```python
from build123d import *

# Parameters (mm, degrees)
SKETCH_W        = 57
SKETCH_H        = 34
PAD_DEPTH       = 15
SKETCH001_W     = 53.5
SKETCH001_H     = 30.5
POCKET_DEPTH    = 2
SKETCH002_W     = 10
SKETCH002_H     = 15.25
POCKET001_DEPTH = 10.7
SKETCH003_W     = 10
SKETCH003_H     = 4.2
POCKET002_DEPTH = 0.45
SKETCH004_W     = 13
SKETCH004_H     = 11.05
POCKET003_DEPTH = 4.9
SKETCH005_W     = 8.9
SKETCH005_H     = 4
POCKET004_DEPTH = 3.6
SKETCH006_W     = 4.5
SKETCH006_H     = 2.4
POCKET005_DEPTH = 2.1
SKETCH007_W     = 51
SKETCH007_H     = 30.5
POCKET006_DEPTH = 2.5


with BuildPart() as part:
    # Sketch → Pad (new body)
    with BuildSketch(Plane.XY):
        Rectangle(SKETCH_W, SKETCH_H)
    extrude(amount=PAD_DEPTH)

    # Sketch001 (on Face6 of Pad) → Pocket (cut)
    with BuildSketch(Plane.XY.offset(15)):
        Rectangle(SKETCH001_W, SKETCH001_H)
    extrude(amount=-POCKET_DEPTH, mode=Mode.SUBTRACT)

    # Sketch002 (on Face11 of Pocket) → Pocket001 (cut)
    with BuildSketch(Plane.XY.offset(13)):
        with Locations((-19.75, 7.625)):
            Rectangle(SKETCH002_W, SKETCH002_H)
        with Locations((20.2, 7.625)):
            Rectangle(SKETCH002_W, SKETCH002_H)
    extrude(amount=-POCKET001_DEPTH, mode=Mode.SUBTRACT)

    # Sketch003 (on Face18 of Pocket001) → Pocket002 (cut)
    with BuildSketch(Plane.XY.offset(2.3)):
        with Locations((-19.75, 13.15)):
            Rectangle(SKETCH003_W, SKETCH003_H)
        with Locations((20.2, 13.15)):
            Rectangle(SKETCH003_W, SKETCH003_H)
    extrude(amount=-POCKET002_DEPTH, mode=Mode.SUBTRACT)

    # Sketch004 (on Face10 of Pocket002) → Pocket003 (cut)
    with BuildSketch(Plane.XY.offset(13)):
        with Locations((-7.8, 9.725)):
            Rectangle(SKETCH004_W, SKETCH004_H)
        with Locations((7.8, 9.725)):
            Rectangle(SKETCH004_W, SKETCH004_H)
    extrude(amount=-POCKET003_DEPTH, mode=Mode.SUBTRACT)

    # Sketch005 (on Face10 of Pocket003) → Pocket004 (cut)
    with BuildSketch(Plane.XY.offset(13)):
        with Locations((10.55, -0.3)):
            Rectangle(SKETCH005_W, SKETCH005_H)
    extrude(amount=-POCKET004_DEPTH, mode=Mode.SUBTRACT)

    # Sketch006 (on Face36 of Pocket004) → Pocket005 (cut)
    with BuildSketch(Plane.XY.offset(9.4)):
        with Locations((10.5, -0.3)):
            Rectangle(SKETCH006_W, SKETCH006_H)
    extrude(amount=-POCKET005_DEPTH, mode=Mode.SUBTRACT)

    # Sketch007 (on Face11 of Pocket005) → Pocket006 (cut)
    with BuildSketch(Plane.XY.offset(13)):
        Rectangle(SKETCH007_W, SKETCH007_H)
    extrude(amount=-POCKET006_DEPTH, mode=Mode.SUBTRACT)


solid = part.part
```
Geometry check sheet. Reference: the model listing, model coordinates, mm. A direction names the side the tool comes from. Round coordinates to 2 decimals unless told otherwise and drop trailing zeros. Order: outer loops, then holes, each group sorted by start corner. A loop starts at its lowest first (then second) coordinate and runs counter-clockwise, first axis right, second up. Notation, with made-up numbers: M 69,70.25 L 119,70.25 A14 ccw 119,86.25 Z; hole C 77.5,-6.5 d9. An arc over 180 degrees is marked long. Answer as CSV lines item,"result".
1) Sectioned sample at A-A on z = 3.25. Record the cut outline in (x, y), and give its area (3 significant figures).
Entries:
outline,"M -28.5,-17 L 28.5,-17 L 28.5,17 L -28.5,17 Z; hole M -24.75,0 L -14.75,0 L -14.75,15.25 L -24.75,15.25 Z; hole M 15.2,0 L 25.2,0 L 25.2,15.25 L 15.2,15.25 Z"
area,"1,630 mm2"
2) Gauge pin test, flat ends, axial feed: pin 1 Ø2 at (x, y) = (-21.5, 13.5) entering from +Z; pin 2 Ø1 at (x, y) = (26, 7.5) entering from +Z; pin 3 Ø5 at (x, y) = (0.5, 3) entering from +Z. Record the tip position at first contact, or that the pin passes through.
Entries:
pin 1,"z = 1.85"
pin 2,"z = 13"
pin 3,"z = 10.5"
3) Thickness scan on probe 1 along Y at (x, z) = (14, 10.25); probe 2 along X at (y, z) = (5.5, 7); probe 3 along X at (y, z) = (10.5, 11). Record the ranges inside material, lowest first. Write a range as [from, to].
Entries:
probe 1,"[-17, -2.3], [1.7, 4.2], [15.25, 17]"
probe 2,"[-28.5, -24.75], [-14.75, 15.2], [25.2, 28.5]"
probe 3,"[-28.5, -25.5], [25.5, 28.5]"
4) Mould release check, pull along Y, two halves, no side actions. Record for faces 3 (the face through (0, 0, 0)), 4 (the face through (0, -17, 7)), 5 (the face through (12.75, 0, 8)): +Y half, -Y half, draft (parallel to the pull), parting line (faces both ways), or undercut.
Entries:
face 3,"draft"
face 4,"-Y half"
face 5,"undercut"
5) Sectioned sample at B-B on z = 14. Record the cut outline in (x, y), and give its area (3 significant figures).
Entries:
outline,"M -28.5,-17 L 28.5,-17 L 28.5,17 L -28.5,17 Z; hole M -26.75,-15.25 L 26.75,-15.25 L 26.75,15.25 L -26.75,15.25 Z"
area,"306 mm2"
6) Sectioned sample at D-D on x = -4.5. Record the cut outline in (y, z).
Entries:
outline,"M -17,0 L 17,0 L 17,15 L 15.25,15 L 15.25,8.1 L 4.2,8.1 L 4.2,10.5 L -15.25,10.5 L -15.25,15 L -17,15 Z"
7) Tool access check on faces 1 (the face through (26.75, 0, 14)), 2 (the face through (28.5, 0, 7)). Record the directions out of +Z, -Z, +X, -X, +Y, -Y that give a thin tool (end or side, any length) a straight path to the whole face; none if there is none.
Entries:
face 1,"+Z"
face 2,"+Z, -Z, +X, +Y, -Y"
8) Sectioned sample at C-C on y = 14. Record the cut outline in (x, z).
Entries:
outline,"M -28.5,0 L 28.5,0 L 28.5,15 L 26.75,15 L 26.75,13 L 25.5,13 L 25.5,10.5 L 25.2,10.5 L 25.2,1.85 L 15.2,1.85 L 15.2,10.5 L 14.3,10.5 L 14.3,8.1 L 1.3,8.1 L 1.3,10.5 L -1.3,10.5 L -1.3,8.1 L -14.3,8.1 L -14.3,10.5 L -14.75,10.5 L -14.75,1.85 L -24.75,1.85 L -24.75,10.5 L -25.5,10.5 L -25.5,13 L -26.75,13 L -26.75,15 L -28.5,15 Z"
